Source: three-view drawing plus pictorial views. Frame: mm from the lowest corner of the part. A direction names the side the tool comes from. Give positions to 0.01 mm unless a question says otherwise; leave off trailing zeros. Order: outer loops, then holes, each group sorted by start corner. A loop starts at its lowest first (then second) coordinate and runs counter-clockwise, first axis right, second up. Notation, with made-up numbers: M 54,19 L 78,19 A31 ccw 78,50 Z; hole C 2,35 d11. An arc over 180 degrees is marked long. Use CSV: the item, a comma, the result in double quotes. Start each with the question number.
1. Section query D-D, the plane x = 42. Return the cut outline in (y, z), plus the area to 3 significant figures.
2. Section query C-C, the plane y = 36. Return the cut outline in (x, z) (1 decimal).
3. Pin query (flat end, axial travel): P1, Ø14, axis at x = 59, y = 41.5, coming from the +Z side; P2, Ø14, axis at x = 54.5, y = 7, coming from the +Z side (1 decimal); P3, Ø2, axis at x = 36.5, y = 28, coming from the -Z side; P4, Ø3, axis at y = 36, z = 66.5, coming from the -X side. Return the tip coordinate at first contact, or that it passes through.
4. Reachability of the marked faces 4, 5, 6, 7 and 8 from +Z, -Z, +X, -X, +Y, -Y: full face, straight path, thin tool, end or side. Return the list, or none.
5. Line query: line 1 along Y through (x, z) = (34, 25.4); line 2 along X through (y, z) = (39.5, 34); line 3 along Z through (x, y) = (25, 25). Output: solid intervals per line, ascending. Write a range as [from, to].
6. Mould query, pull axis X, two halves, no side actions, for the marked faces 1, 2 and 3. Classes: released by +X, released by -X, zero draft, split by the parting line, or undercut.
7. Section query B-B, the plane z = 21. Return the cut outline in (x, y) (1 decimal), plus the area to 3 significant figures.
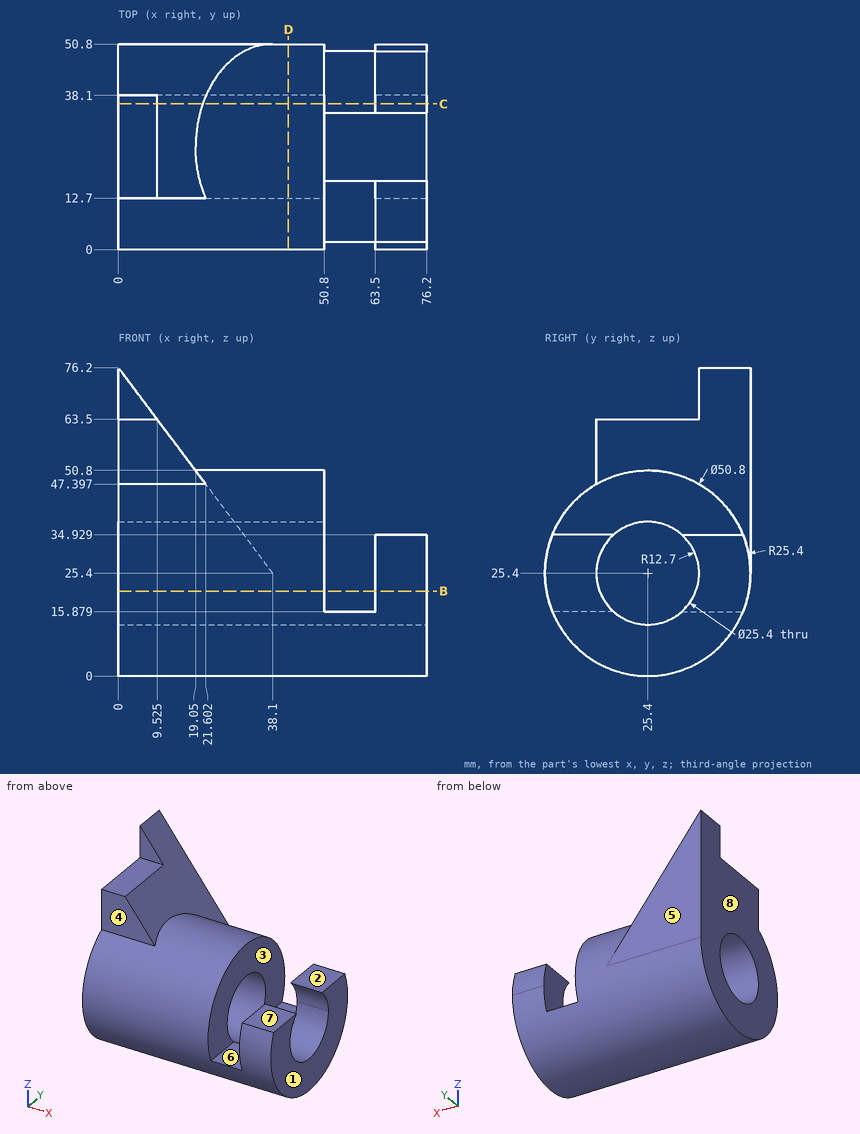
Result set:
1,outline,"C 25.4,25.4 d50.8; hole C 25.4,25.4 d25.4"
1,area,"1,520 mm2"
2,outline,"M 0,2.3 L 76.2,2.3 L 76.2,18.4 L 63.5,18.4 L 63.5,15.9 L 50.8,15.9 L 50.8,18.4 L 0,18.4 Z; M 0,32.4 L 50.8,32.4 L 50.8,48.5 L 20.8,48.5 L 9.5,63.5 L 0,63.5 Z; M 63.5,32.4 L 76.2,32.4 L 76.2,34.9 L 63.5,34.9 Z"
3,P1,"z = 34.93"
3,P2,"z = 47.5"
3,P3,"z = 0.05"
3,P4,"through"
4,face 4,"+Z, +X, -X, -Y"
4,face 5,"+Z, -Z, +X, -X, +Y"
4,face 6,"+Z, +Y, -Y"
4,face 7,"+Z, +X, +Y, -Y"
4,face 8,"+Z, -Z, -X, +Y, -Y"
5,line 1,"[0, 12.7], [38.1, 50.8]"
5,line 2,"[0, 50.8], [63.5, 76.2]"
5,line 3,"[0, 12.71], [38.09, 50.8]"
6,face 1,"released by +X"
6,face 2,"zero draft"
6,face 3,"undercut"
7,outline,"M 0,0.4 L 50.8,0.4 L 50.8,13.5 L 0,13.5 Z; M 0,37.3 L 50.8,37.3 L 50.8,50.4 L 0,50.4 Z; M 63.5,0.4 L 76.2,0.4 L 76.2,13.5 L 63.5,13.5 Z; M 63.5,37.3 L 76.2,37.3 L 76.2,50.4 L 63.5,50.4 Z"
7,area,"1,660 mm2"
